Source: CAD feature listing. Evaluate the final solid. Frame: model axes, mm. Face numbers are marked on the shaded views. A direction names the side the tool comes from. Round coordinates to 2 decimals unless told otherwise and drop trailing zeros. Order: outer loops, then holes, each group sorted by start corner. A loop starts at its lowest first (then second) coordinate and runs counter-clockwise, first axis right, second up. Notation, with made-up numbers: (-22, 8) - (3, 8) arc R19 ccw to (3, 21) - close; hole circle Ø2 at (82, 62.25). An arc over 180 degrees is marked (long way). Put each result on its own line as item: value. Start each with the question number.
1) Section A-A on y = 28. Output: boundary loops of the cut face in (x, z), then the cut area to 3 significant figures.
2) Section D-D on z = 22.5. Output: boundary loops of the cut face in (x, y).
3) Section B-B on x = 15. State how many separate pieces and enclosed holes the cut face has, then the cut area to 3 significant figures.
4) Contact query for flat-ended pins moving along their axis: P1, Ø8, axis at x = -15, z = 60, coming from the +Y side; P2, Ø4, axis at x = -4, z = -26.5, coming from the +Y side; P3, Ø2, axis at x = -11, z = -23, coming from the +Y side. Output: stop coordinate, or through.
5) Access query for the marked faces 5, 6 and 7. Directions: +Z, -Z, +X, -X, +Y, -Y. A direction counts if a zero-diameter tool reaches every point of the face in a straight line with its end or side. Return the directions, or none.
6) Mould query, pull axis Z, two halves, no side actions, for the marked faces 1, 2, 3 and 4. Classes: +Z half, -Z half, draft (parallel to the pull), parting line (faces both ways), or undercut.
7) Section C-C on z = 60. Output: boundary loops of the cut face in (x, y).
8) Line query: probe 1 along X at (y, z) = (4, 60); probe 2 along Z at (x, y) = (21, 20); probe 3 along Y at (x, z) = (-17, -40). Output: solid intervals per line, ascending. Write a range as [from, to].
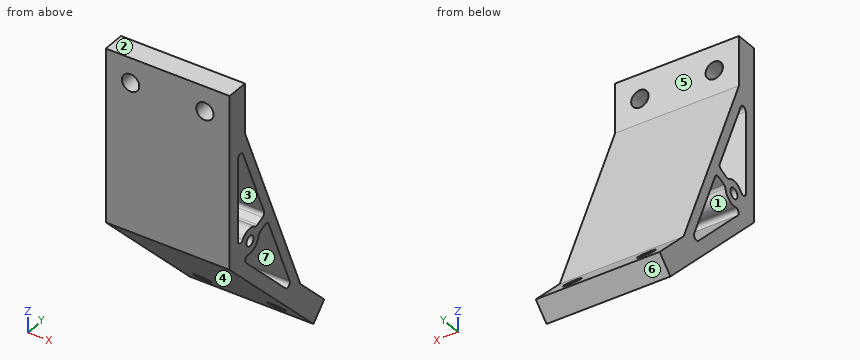
```python
from build123d import *

# Parameters (mm, degrees)
BOSS_EXTRUDE1_DEPTH      = 25
BOSS_EXTRUDE1_DEPTH_BACK = 25
SKETCH1_R                = 2.1
SKETCH2_R                = 3.5
CUT_EXTRUDE1_DEPTH       = 9
SKETCH3_R                = 3.5
CUT_EXTRUDE2_DEPTH       = 9


with BuildPart() as part:
    # Sketch1 → Boss-Extrude1 (new, two sides: drawn at the far end of the back side and taken through both)
    with BuildSketch(Plane(origin=(0, 0, 0), x_dir=(0, 0, -1), z_dir=(1, 0, 0)).offset(-BOSS_EXTRUDE1_DEPTH_BACK)):
        Polygon((-70, 0), (0, 0), (49.497474683, 49.497474683), (43.133513652, 55.861435714), (28.991378029, 41.71930009), (-49.991379635, 9), (-70, 9), align=None)
        with Locations((-4.970562748, 12)):
            Circle(SKETCH1_R, mode=Mode.SUBTRACT)
        with BuildLine():
            Line((-6.551793043, 21.043679481), (-5.264121815, 17.934966139))
            ThreePointArc((-5.264121815, 17.934966139), (-4.812340099, 17.335290392), (-4.126543478, 17.029675086))
            ThreePointArc((-4.126543478, 17.029675086), (-0.768310337, 14.889822601), (0.028067769, 10.988222878))
            ThreePointArc((0.028067769, 10.988222878), (0.788934633, 9.368950353), (2.558913388, 9.6299812))
            Line((2.558913388, 9.6299812), (25.924897249, 32.995965061))
            ThreePointArc((25.924897249, 32.995965061), (26.111441495, 34.889980582), (24.290211928, 35.442444531))
            Line((24.290211928, 35.442444531), (-5.739998892, 23.003523928))
            ThreePointArc((-5.739998892, 23.003523928), (-6.551793043, 22.191729778), (-6.551793043, 21.043679481))
        make_face(mode=Mode.SUBTRACT)
        with BuildLine():
            Line((-41.755939666, 5.002860881), (-8.61897952, 5.000000011))
            ThreePointArc((-8.61897952, 5.000000011), (-7.181021866, 6.072446959), (-7.79931621, 7.756364052))
            ThreePointArc((-7.79931621, 7.756364052), (-9.986482643, 11.077634818), (-9.123891859, 14.959705611))
            ThreePointArc((-9.123891859, 14.959705611), (-8.855063072, 15.660739707), (-8.959639945, 16.40423241))
            Line((-8.959639945, 16.40423241), (-10.247311173, 19.512945751))
            ThreePointArc((-10.247311173, 19.512945751), (-11.013696575, 20.305047115), (-12.114513279, 20.35957911))
            Line((-12.114513279, 20.35957911), (-42.237227636, 7.885876778))
            ThreePointArc((-42.237227636, 7.885876778), (-43.142866755, 6.253009403), (-41.755939666, 5.002860881))
        make_face(mode=Mode.SUBTRACT)
    extrude(amount=BOSS_EXTRUDE1_DEPTH + BOSS_EXTRUDE1_DEPTH_BACK)

    # Sketch2 → Cut-Extrude1 (cut)
    with BuildSketch(Plane(origin=(0, 0, 0), x_dir=(1, 0, 0), z_dir=(0, 1, 0))):
        with Locations(Location((-15, -60, 0), (0, 0, 270))):
            Circle(SKETCH2_R)
    extrude(amount=CUT_EXTRUDE1_DEPTH, mode=Mode.SUBTRACT)

    # Sketch3 → Cut-Extrude2 (cut)
    with BuildSketch(Plane(origin=(0, 0, 0), x_dir=(1, 0, 0), z_dir=(0, 1, 0))):
        with Locations(Location((15, -60, 0), (0, 0, 270))):
            Circle(SKETCH3_R)
    extrude(amount=CUT_EXTRUDE2_DEPTH, mode=Mode.SUBTRACT)

    # Sketch4 → Cut-Revolve1 (revolve, cut)
    with BuildSketch(Plane(origin=(15, 0, 0), x_dir=(0, 0, -1), z_dir=(1, 0, 0)), mode=Mode.PRIVATE) as cut_revolve1_sk:
        Polygon((36.062445841, 48.790367902), (38.537319575, 51.265241636), (44.901280605, 44.901280605), (42.426406871, 42.426406871), align=None)
    revolve(cut_revolve1_sk.sketch.rotate(Axis((15, 42.426406871, -42.426406871), (0, 0.7071067811865476, 0.7071067811865476)), 180), axis=Axis((15, 42.426406871, -42.426406871), (0, 0.7071067811865476, 0.7071067811865476)), mode=Mode.SUBTRACT)

    # Sketch5 → Cut-Revolve2 (revolve, cut)
    with BuildSketch(Plane(origin=(-15, 0, 0), x_dir=(0, 0, -1), z_dir=(1, 0, 0)), mode=Mode.PRIVATE) as cut_revolve2_sk:
        Polygon((36.062445841, 48.790367902), (38.537319575, 51.265241636), (44.901280605, 44.901280605), (42.426406871, 42.426406871), align=None)
    revolve(cut_revolve2_sk.sketch.rotate(Axis((-15, 42.426406871, -42.426406871), (0, 0.7071067811865476, 0.7071067811865476)), 180), axis=Axis((-15, 42.426406871, -42.426406871), (0, 0.7071067811865476, 0.7071067811865476)), mode=Mode.SUBTRACT)


solid = part.part
```
Answer sheet:
1. outline: (-25, -28) - (25, -28) - (25, -20.93) - (-25, -20.93) - close; (-25, -6.32) - (25, -6.32) - (25, 4.13) - (-25, 4.13) - close
1. area: 876 mm^2
2. outline: (-25, 0) - (25, 0) - (25, 5) - (-25, 5) - close; (-25, 16.06) - (25, 16.06) - (25, 20.39) - (-25, 20.39) - close
3. separate pieces: 3
3. enclosed holes: 3
3. area: 1,200 mm^2
4. P1: y = 9
4. P2: y = 41.52
4. P3: y = 39.65
5. face 5: +Z, +X, -X, +Y
5. face 6: -Z, +X, -X, +Y
5. face 7: +X, -X
6. face 1: undercut
6. face 2: +Z half
6. face 3: undercut
6. face 4: -Z half
7. outline: (-25, 0) - (-18.5, 0) - (-18.5, 9) - (-25, 9) - close; (-11.5, 0) - (11.5, 0) - (11.5, 9) - (-11.5, 9) - close; (18.5, 0) - (25, 0) - (25, 9) - (18.5, 9) - close
8. probe 1: [-25, -18.5], [-11.5, 11.5], [18.5, 25]
8. probe 2: [-20, -12.93], [6.12, 10.57], [12.98, 23.44]
8. probe 3: [40, 40.79], [48.91, 52.73]
